Can you work these out from the model? Positions are in its coordinate system, mm. Give positions to 0.01 mm unless a question says otherwise; leave off trailing zeros. Order: outer loops, then holes, each group sorted by start corner. A loop starts at its lowest first (then second) coordinate and runs counter-clockwise, first axis right, second up. Notation, with made-up numbers: (83.25, 43) - (125.25, 43) arc R13 ccw to (125.25, 65) - close; hole circle Ø10 at (19, -36.75). An arc over 180 degrees is marked (long way). Answer as CSV lines item,"result".
```python
from build123d import *

# Parameters (mm, degrees)
SKETCH2_W           = 250
SKETCH2_H           = 250
BOSS_EXTRUDE1_DEPTH = 3.175
SKETCH3_W           = 8.6
SKETCH3_H           = 15.35
CUT_EXTRUDE1_DEPTH  = 10
SKETCH10_W          = 45
SKETCH10_H          = 3.175
BOSS_EXTRUDE2_DEPTH = 12.5
SKETCH11_W          = 45
SKETCH11_H          = 3.175
BOSS_EXTRUDE3_DEPTH = 12.5
SKETCH13_W          = 45
SKETCH13_H          = 3.175
BOSS_EXTRUDE4_DEPTH = 12.5
SKETCH14_W          = 45
SKETCH14_H          = 3.175
BOSS_EXTRUDE5_DEPTH = 12.5
M3_TAPPED_HOLE1_D   = 2.5
SKETCH21_R          = 1.25
CUT_EXTRUDE2_DEPTH  = 10


with BuildPart() as part:
    # Sketch2 → Boss-Extrude1 (new body)
    with BuildSketch(Plane(origin=(0, 0, 0), x_dir=(1, 0, 0), z_dir=(0, 1, 0))):
        Rectangle(SKETCH2_W, SKETCH2_H)
    extrude(amount=BOSS_EXTRUDE1_DEPTH)

    # Sketch3 → Cut-Extrude1 (cut)
    with BuildSketch(Plane(origin=(0, 3.175, 0), x_dir=(1, 0, 0), z_dir=(0, 1, 0))):
        with Locations((-43.75, 35.675)):
            Rectangle(SKETCH3_W, SKETCH3_H)
        with Locations((-43.75, -35.675)):
            Rectangle(SKETCH3_W, SKETCH3_H)
        with Locations((43.75, -35.675)):
            Rectangle(SKETCH3_W, SKETCH3_H)
        with Locations((43.75, 35.675)):
            Rectangle(SKETCH3_W, SKETCH3_H)
    extrude(amount=-CUT_EXTRUDE1_DEPTH, mode=Mode.SUBTRACT)

    # Sketch10 → Boss-Extrude2 (add)
    with BuildSketch(Plane(origin=(0, 0, -125), x_dir=(-1, 0, 0), z_dir=(0, 0, -1))):
        with Locations((0, 1.5875)):
            Rectangle(SKETCH10_W, SKETCH10_H)
    extrude(amount=BOSS_EXTRUDE2_DEPTH)

    # Sketch11 → Boss-Extrude3 (add)
    with BuildSketch(Plane.ZY.offset(125)):
        with Locations((0, 1.5875)):
            Rectangle(SKETCH11_W, SKETCH11_H)
    extrude(amount=BOSS_EXTRUDE3_DEPTH)

    # Sketch13 → Boss-Extrude4 (add)
    with BuildSketch(Plane.XY.offset(125)):
        with Locations((0, 1.5875)):
            Rectangle(SKETCH13_W, SKETCH13_H)
    extrude(amount=BOSS_EXTRUDE4_DEPTH)

    # Sketch14 → Boss-Extrude5 (add)
    with BuildSketch(Plane(origin=(125, 0, 0), x_dir=(0, 0, -1), z_dir=(1, 0, 0))):
        with Locations((0, 1.5875)):
            Rectangle(SKETCH14_W, SKETCH14_H)
    extrude(amount=BOSS_EXTRUDE5_DEPTH)

    # M3 Tapped Hole1 (through all)
    with Locations(Plane(origin=(-115, 3.175, -115), x_dir=(0, 0, 1), z_dir=(0, 1, 0))):
        with Locations((0, 0)):
            Hole(M3_TAPPED_HOLE1_D / 2)

    # Sketch21 → Cut-Extrude2 (cut)
    with BuildSketch(Plane(origin=(0, 3.175, 0), x_dir=(1, 0, 0), z_dir=(0, 1, 0))):
        with Locations((115, 115)):
            Circle(SKETCH21_R)
        with Locations((115, -115)):
            Circle(SKETCH21_R)
        with Locations((-115, -115)):
            Circle(SKETCH21_R)
    extrude(amount=-CUT_EXTRUDE2_DEPTH, mode=Mode.SUBTRACT)


solid = part.part
```
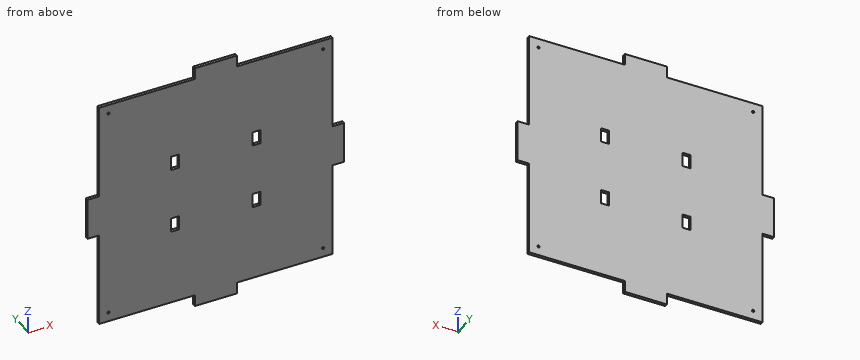
1) I'm going to push flat-ended pins straight in: P1, Ø1.6, axis at x = -44.5, y = 1.5, coming from the -Z side; P2, Ø1.6, axis at x = 130.5, y = 2, coming from the +Z side; P3, Ø1.6, axis at y = 1, z = -32.5, coming from the -X side; P4, Ø1.5, axis at x = -115, z = -115, coming from the +Y side. Where does each tip first touch, or does it pass through?
Answer block:
P1,"z = -125"
P2,"z = 22.5"
P3,"x = -125"
P4,"through"
2) I need wall thicknesses on line 1 along X through (y, z) = (0.4, 31); line 2 along X through (y, z) = (1.5, -115). Which ranges of each line are inside material? Lowest first, please. Write a range as [from, to].
Answer block:
line 1,"[-125, -48.05], [-39.45, 39.45], [48.05, 125]"
line 2,"[-125, -116.25], [-113.75, 113.75], [116.25, 125]"
3) I want a section at B-B on x = -70.5. Write out the boundary of the cut face in (y, z) (3 decimals).
Answer block:
outline,"(0, -125) - (3.175, -125) - (3.175, 125) - (0, 125) - close"
4) I want a section at C-C on z = 69.5. Write out the boundary of the cut face in (x, y) (3 decimals), plus the area to 3 significant figures.
Answer block:
outline,"(-125, 0) - (125, 0) - (125, 3.175) - (-125, 3.175) - close"
area,"794 mm2"
5) I want a section at A-A on y = 0.85. Count the separate pieces of the cut face and the enclosed holes in it, plus the area to 3 significant figures.
Answer block:
separate pieces,"1"
enclosed holes,"8"
area,"64,200 mm2"
